Autodesk Inventor part; units mm, degrees
ref_plane "YZ Plane" through (0, 0, 0) normal (1, 0, 0) x (0, 1, 0)
ref_plane "XZ Plane" through (0, 0, 0) normal (0, 1, 0) x (-1, 0, 0)
ref_plane "XY Plane" through (0, 0, 0) normal (0, 0, 1) x (1, 0, 0)
sketch "Sketch1" plane through (0, 0, 0) normal (0, 1, 0) x (-1, 0, 0)
  circle A0 centre (18.5, 28) radius 23.85
  circle A1 centre (37, -23.25) radius 13.85
  circle A2 centre (-35, -38.75) radius 13.85
  circle A3 centre (-30.9, 25.8) radius 13.85
  circle A4 centre (0, -23.25) radius 13.85
  line L0 (56.25, 58.25) -> (-56.25, 58.25)
  line L1 (-56.25, -58.25) -> (56.25, -58.25)
  line L2 (0, -105.9299) -> (0, 123.2086) construction
  line L3 (-76.4777, -38.75) -> (-5.35, -38.75) construction
  line L4 (-123.5447, -23.25) -> (82.5572, -23.25) construction
  line L5 (56.25, -58.25) -> (56.25, 58.25)
  line L6 (56.25, 58.25) -> (56.25, -58.25)
  line L7 (-56.25, 58.25) -> (-56.25, -58.25)
  line L8 (100.0459, 28) -> (-13.85, 28) construction
  line L9 (-9.7154, 25.8) -> (-68.4996, 25.8) construction
  line L10 (18.5, 82.6038) -> (18.5, -4.654) construction
  line L11 (-30.9, 82.6038) -> (-30.9, 8.6393) construction
  line L12 (-46.6436, -58.25) -> (-56.25, -58.25) construction
  line L13 (-56.25, -58.25) -> (-56.25, -31.25) construction
  line L14 (-56.25, -31.25) -> (-46.6436, -31.25) construction
  line L15 (-46.6436, -31.25) -> (-46.6436, -58.25) construction
  line L16 (56.25, -58.25) -> (48.3059, -58.25) construction
  line L17 (48.3059, -58.25) -> (48.3059, -31.25) construction
  line L18 (48.3059, -31.25) -> (56.25, -31.25) construction
  line L19 (56.25, -31.25) -> (56.25, -58.25) construction
  point P0 (0, 0)
  point P1 (0, 0)
  dimension "d1" = 27.7
  dimension "d2" = 27.7
  dimension "d0" = 47.7
  dimension "d3" = 27.7
  dimension "d4" = 27.7
  dimension "d7" = 37
  dimension "d9" = 30.9
  dimension "d10" = 19.5
  dimension "d11" = 35
  dimension "d12" = 35
  dimension "d13" = 25.8
  dimension "d14" = 28
  dimension "d15" = 56.25
  dimension "d16" = 58.25
  dimension "d17" = 116.5
  dimension "d18" = 112.5
  dimension "d19" = 18.5
  dimension "d20" = 32.45
  dimension "d31" = 27
  dimension "d32" = 9.6064
  dimension "d33" = 27
  dimension "d34" = 7.9441
extrude "Extrusion1" add sketch "Sketch1" along normal blind 5
sketch "Sketch2" plane through (0, 5, 0) normal (0, 1, 0) x (1, 0, 0)
  line L0 (-56.25, 58.25) -> (-56.25, -58.25)
  line L1 (-56.25, -58.25) -> (56.25, -58.25)
  line L2 (56.25, -58.25) -> (56.25, 58.25)
  line L3 (56.25, 58.25) -> (-56.25, 58.25)
  circle A0 centre (0, 23.25) radius 13.85
  circle A1 centre (30.9, -25.8) radius 13.85
  circle A2 centre (35, 38.75) radius 13.85
  circle A3 centre (-37, 23.25) radius 13.85
  circle A4 centre (-18.5, -28) radius 23.85
  line L4 (-56.25, 58.25) -> (-56.25, -58.25)
  line L5 (-56.25, 23.25) -> (15.75, 23.25)
  line L6 (19.75, 38.75) -> (56.25, 38.75)
  line L7 (56.25, -58.25) -> (56.25, 58.25)
  line L8 (17.75, 25.25) -> (17.75, 36.75)
  arc A5 (15.75, 23.25) -> (17.75, 25.25) centre (15.75, 25.25) ccw
  arc A6 (19.75, 38.75) -> (17.75, 36.75) centre (19.75, 36.75) ccw
  point P0 (0, 0)
  point P1 (17.75, 23.25)
  point P2 (17.75, 38.75)
  point P3 (48.85, 38.75)
  point P4 (21.15, 38.75)
  point P5 (13.85, 23.25)
  point P6 (-13.85, 23.25)
  point P7 (-23.15, 23.25)
  point P8 (-50.85, 23.25)
  dimension "d23" = 74
  dimension "d25" = 38.5
  dimension "d26" = 2
  dimension "d27" = 35
  dimension "d28" = 19.5
extrude "Extrusion2" cut sketch "Sketch2" against normal through all contours L5 A3 A0 A5 L8 A6 L6 A2 L2 L1 L0
properties part number "Top Bottle Back"
CAD build for the part. Positions are in the model's coordinates, mm. A direction names the side the tool comes from. Coordinates: 2 decimals unless noted, no trailing zeros. Write each loop counter-clockwise with the first axis right and the second up, starting at its lowest first coordinate (ties: lowest second). Pieces come first, ordered by that corner, then holes.
(1) 3-axis set-ups, long thin cutter, end or side, ignore diameter. For faces 1 (the face through (-0.305, 2.465, -37.097)), 2 (the face through (17.75, 3, -31)): which of +Z, -Z, +X, -X, +Y, -Y reach the whole face in a straight line?
(2) Cut at B-B, the plane z = -41. List the corners of the cut face in (x, y).
(3) Cut at D-D, the plane x = 0. List the corners of the cut face in (y, z), and give its area (3 significant figures).
(4) Cut at A-A, the plane z = -29. List the corners of the cut face in (x, y).
(5) Flat gauge pin, fed straight in: pin 1 (1 mm diameter, centred on y = 2, z = -32, fed in from +X). Where does the tip first touch, or does it go through?
(6) Cut at C-C, the plane y = 2.65. List the corners of the cut face in (x, z), and give its area (3 significant figures).
(7) Drill centre lines: probe 1 along X at (y, z) = (3.35, -30.5); probe 2 along X at (y, z) = (0.35, -27); probe 3 along X at (y, z) = (4, -39). Where is each one in solid material? Low to high.
(8) Two-plate mould, pull along X, no slides. Class faces 3 (the face through (34.695, 2.465, -52.597)), 4 (the face through (-56.25, 2, -41)), 5 (the face through (-12, 0, -44)): +X half, -X half, draft (parallel to the pull), parting line (faces both ways), or undercut.
Geometry says:
1. face 1: +Z, +Y, -Y
1. face 2: +Z, +X, +Y, -Y
2. outline: (-56.25, 0) - (21.33, 0) - (21.33, 5) - (-56.25, 5) - close; (48.67, 0) - (56.25, 0) - (56.25, 5) - (48.67, 5) - close
3. outline: (0, -58.25) - (5, -58.25) - (5, -37.1) - (0, -37.1) - close
3. area: 106 mm2
4. outline: (-56.25, 0) - (-49.6, 0) - (-49.6, 5) - (-56.25, 5) - close; (-24.4, 0) - (-12.6, 0) - (-12.6, 5) - (-24.4, 5) - close; (12.6, 0) - (17.75, 0) - (17.75, 5) - (12.6, 5) - close
5. pin 1: stops at x = 17.75
6. outline: (-56.25, -58.25) - (56.25, -58.25) - (56.25, -38.75) - (48.85, -38.75) arc R13.85 cw to (21.15, -38.75) - (19.75, -38.75) arc R2 cw to (17.75, -36.75) - (17.75, -25.25) arc R2 ccw to (15.75, -23.25) - (13.85, -23.25) arc R13.85 cw to (-13.85, -23.25) - (-23.15, -23.25) arc R13.85 cw to (-50.85, -23.25) - (-56.25, -23.25) - close
6. area: 2,440 mm2
7. probe 1: x = -56.25 to -48.8, -25.2 to -11.8, 11.8 to 17.75
7. probe 2: x = -56.25 to -50.33, -23.67 to -13.33, 13.33 to 17.75
7. probe 3: x = -56.25 to 21.15, 48.85 to 56.25
8. face 3: undercut
8. face 4: -X half
8. face 5: draft
